Design review of the part shown in the three views and the two pictorial views. Dimensions are in mm from the part's minimum x, y and z. Give positions to 0.01 mm unless a question says otherwise; leave off trailing zeros. Loops run counter-clockwise (first coordinate to the right, second up) from the corner with the lowest first, then second, coordinate; pieces in that order, holes last.
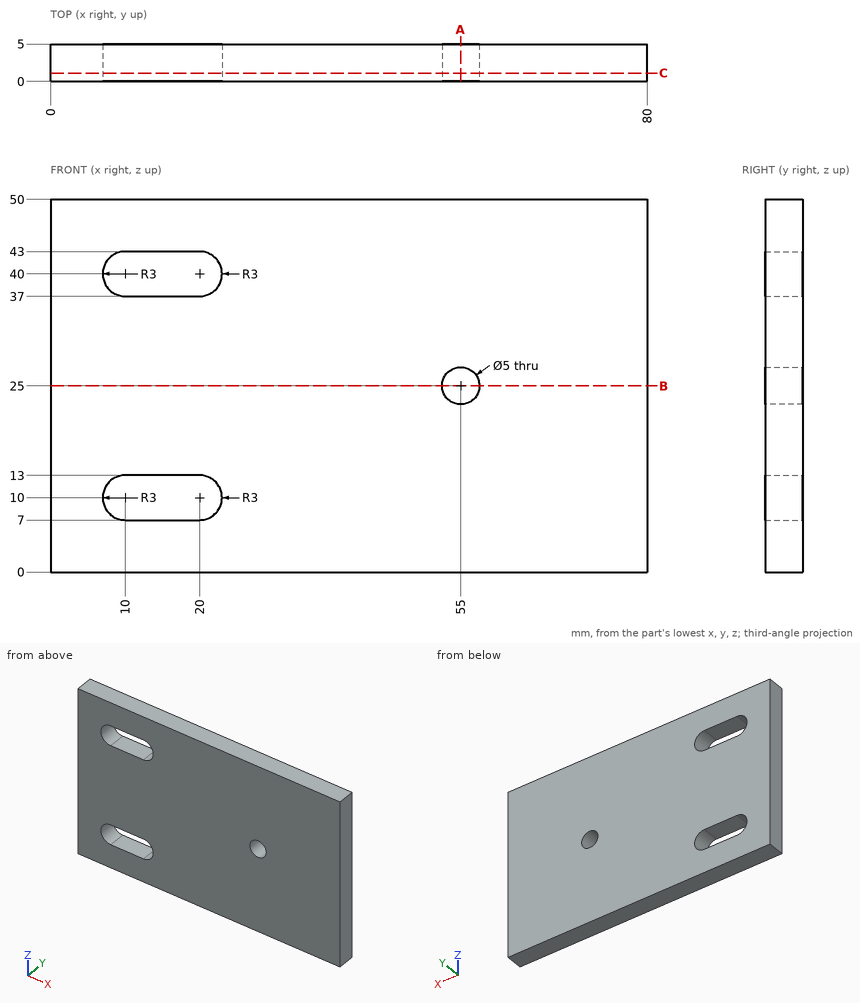
Q1. Take a section at A-A (x = 55). Give the boundary of the cut face in (y, z), plus the area to 3 significant figures.
Results:
outline: (0, 0) - (5, 0) - (5, 22.5) - (0, 22.5) - close; (0, 27.5) - (5, 27.5) - (5, 50) - (0, 50) - close
area: 225 mm2
Q2. Insertion check: pin 1 (1.5 mm diameter, centred on x = 15, y = 1.5, fed in from -Z). The pin has a flat end and moves straight along its axis. Give the tip position at first contact, or say it passes through.
Results:
pin 1: stops at z = 0
Q3. Wall thickness on line 1 (Z direction, x = 15, y = 0.85); line 2 (X direction, y = 3.35, z = 25); line 3 (X direction, y = 4.3, z = 8.5): over which ranges is each line inside the solid? List them lowest first.
Results:
line 1: z = 0 to 7, 13 to 37, 43 to 50
line 2: x = 0 to 52.5, 57.5 to 80
line 3: x = 0 to 7.4, 22.6 to 80
Q4. Take a section at C-C (y = 1.1). Give the boundary of the cut face in (x, z), plus the area to 3 significant figures.
Results:
outline: (0, 0) - (80, 0) - (80, 50) - (0, 50) - close; hole (10, 7) - (20, 7) arc R3 ccw to (20, 13) - (10, 13) arc R3 ccw to start; hole (10, 37) - (20, 37) arc R3 ccw to (20, 43) - (10, 43) arc R3 ccw to start; hole circle Ø5 at (55, 25)
area: 3,800 mm2
Q5. Take a section at B-B (z = 25). Give the boundary of the cut face in (x, y), plus the area to 3 significant figures.
Results:
outline: (0, 0) - (52.5, 0) - (52.5, 5) - (0, 5) - close; (57.5, 0) - (80, 0) - (80, 5) - (57.5, 5) - close
area: 375 mm2
